```python
from build123d import *

# Parameters (mm, degrees)
BOSS_EXTRUDE1_DEPTH       = 8.2
CUT_EXTRUDE1_DEPTH        = 2.2
SKETCH3_W                 = 6.75
SKETCH3_H                 = 8.2
BOSS_EXTRUDE2_DEPTH       = 4
M2X0_4_TAPPED_HOLE1_D     = 1.6
M2X0_4_TAPPED_HOLE1_DEPTH = 4.7
M2X0_4_TAPPED_HOLE1_TIP   = 0.480688495
F_1_5MM_DOWEL_HOLE1_D     = 1.5
F_1_5MM_DOWEL_HOLE1_DEPTH = 3
F_1_5MM_DOWEL_HOLE1_TIP   = 0.450645464


with BuildPart() as part:
    # Sketch1 → Boss-Extrude1 (new body)
    with BuildSketch(Plane.XY):
        Polygon((0, 0), (6.75, 0), (6.75, 4.788271091), (5.75, 4.788271091), (4.167950223, 6.316038802), (0, 2), align=None)
    extrude(amount=BOSS_EXTRUDE1_DEPTH)

    # Sketch2 → Cut-Extrude1 (cut)
    with BuildSketch(Plane(origin=(-0.999390827, 0.965100503, 0), x_dir=(0.69465837, 0.7193398, 0), z_dir=(-0.7193398, 0.69465837, 0))):
        with BuildLine():
            Line((8.438679601, 0), (8.438679601, -6.2))
            Line((8.438679601, -6.2), (3.438679601, -6.2))
            Line((3.438679601, -6.2), (3.438679601, -6.45))
            ThreePointArc((3.438679601, -6.45), (2.438679601, -7.45), (1.438679601, -6.45))
            Line((1.438679601, -6.45), (1.438679601, 0))
            Line((1.438679601, 0), (8.438679601, 0))
        make_face()
    extrude(amount=-CUT_EXTRUDE1_DEPTH, mode=Mode.SUBTRACT)

    # Sketch3 → Boss-Extrude2 (add)
    with BuildSketch(Plane.XZ):
        with Locations((3.375, 4.1)):
            Rectangle(SKETCH3_W, SKETCH3_H)
    extrude(amount=BOSS_EXTRUDE2_DEPTH)

    # M2x0.4 Tapped Hole1
    with Locations(Plane(origin=(0, -4, 0), x_dir=(-1, 0, 0), z_dir=(0, -1, 0))):
        with Locations((-3.75, -4.1)):
            Hole(M2X0_4_TAPPED_HOLE1_D / 2, depth=M2X0_4_TAPPED_HOLE1_DEPTH)
            with Locations((0, 0, -(M2X0_4_TAPPED_HOLE1_DEPTH + M2X0_4_TAPPED_HOLE1_TIP / 2))):  # 118° drill point
                Cone(0, M2X0_4_TAPPED_HOLE1_D / 2, M2X0_4_TAPPED_HOLE1_TIP, mode=Mode.SUBTRACT)

    # Ø1.5mm Dowel Hole1
    with Locations(Plane(origin=(0, -4, 0), x_dir=(-1, 0, 0), z_dir=(0, -1, 0))):
        with Locations((-3.75, -7.1), (-3.75, -1.1)):
            Hole(F_1_5MM_DOWEL_HOLE1_D / 2, depth=F_1_5MM_DOWEL_HOLE1_DEPTH)
            with Locations((0, 0, -(F_1_5MM_DOWEL_HOLE1_DEPTH + F_1_5MM_DOWEL_HOLE1_TIP / 2))):  # 118° drill point
                Cone(0, F_1_5MM_DOWEL_HOLE1_D / 2, F_1_5MM_DOWEL_HOLE1_TIP, mode=Mode.SUBTRACT)


solid = part.part
```
Design review of the part built by this model. Coordinates are the model's own, in mm. A direction names the side the tool comes from. Give positions to 0.01 mm unless a question says otherwise; leave off trailing zeros. Order: outer loops, then holes, each group sorted by start corner. A loop starts at its lowest first (then second) coordinate and runs counter-clockwise, first axis right, second up. Notation, with made-up numbers: M 21,-15 L 55,-15 A24 ccw 55,0 Z; hole C -10.5,4 d8. An arc over 180 degrees is marked long. One line per question, with ' | ' between items. Start each with the question number.
Q1. Machinability: for faces 4 (the face through (6, 4.788, 4)), 5 (the face through (3, -2.5, 1.1)), 6 (the face through (2.6, -4, 4.2)), which of the approach directions +Z, -Z, +X, -X, +Y, -Y give a long, thin tool a straight path to every point of the face, cutting with its end or side? Answer none if there is none.
Q2. We need section B-B (y = 0). Write out the cut boundary in (x, z), plus the area to 3 significant figures.
Q3. We need section C-C (x = 5.25). Write out the cut boundary in (y, z).
Q4. For L1, parallel to Z at x = 3.75, y = -2.1; L2, parallel to X at y = -2.5, z = 7.1; L3, parallel to X at y = 1.25, z = 2.75, list the stretches that pass through material, from the lowest coordinate up. Write a range as [from, to].
Q5. For pin 1 Ø1.3 at (x, z) = (3.75, 4.1) entering from -Y; pin 2 Ø3 at (x, z) = (1, 3.5) entering from +Y; pin 3 Ø0.8 at (x, z) = (6.5, 6) entering from +Y, all flat-tipped, find the tip position at first contact; note any pin that passes through.
Q6. We need section A-A (y = -1.5). Write out the cut boundary in (x, z), plus the area to 3 significant figures.
Q7. The part is to be moulded in two halves that separate along Z. For faces 1 (the face through (3.587, -2.479, 7.832)), 2 (the face through (0, -1, 4)), 3 (the face through (4, 4, 6.2)), say which applies: +Z half, -Z half, draft (parallel to the pull), parting line (faces both ways), or undercut.
Returned:
1) face 4: +Z, -Z, +X, +Y | face 5: -Y | face 6: +Z, -Z, +X, -X, -Y
2) outline: M 0,0 L 6.75,0 L 6.75,8.2 L 0,8.2 Z; hole C 3.75,4.1 d1.6 | area: 53.3 mm2
3) outline: M -4,0 L 4.27,0 L 4.27,6.2 L 5.27,6.2 L 5.27,8.2 L -4,8.2 Z
4) L1: [0, 0.35], [1.85, 3.3], [4.9, 6.35], [7.85, 8.2] | L2: [0, 3], [4.5, 6.75] | L3: [0, 0.78], [2.33, 6.75]
5) pin 1: y = 0.79 | pin 2: y = 2 | pin 3: y = 4.79
6) outline: M 0,0 L 6.75,0 L 6.75,8.2 L 0,8.2 Z; hole C 3.75,4.1 d1.6; hole C 3.75,1.1 d1.5; hole C 3.75,7.1 d1.5 | area: 49.8 mm2
7) face 1: undercut | face 2: draft | face 3: -Z half
